CAD build for the part. Positions are in the model's coordinates, mm. Round coordinates to 2 decimals unless told otherwise and drop trailing zeros. Loops run counter-clockwise (first coordinate to the right, second up) from the corner with the lowest first, then second, coordinate; pieces in that order, holes last. Notation, with made-up numbers: (-20, -0.75) -> (5, -0.75) arc R28 cw to (5, 32.25) -> close; hole circle Ø3 at (85.25, 25.25). An arc over 180 degrees is marked (long way). Answer as CSV lines item,"result".
```python
from build123d import *

# Parameters (mm, degrees)
SKETCH1_R           = 12.7
SKETCH1_R_2         = 11.7
EXTRUDE_THIN1_DEPTH = 275.4


with BuildPart() as part:
    # Sketch1 → Extrude-Thin1 (new, symmetric)
    with BuildSketch(Plane(origin=(0, 0, 0), x_dir=(0, 0, -1), z_dir=(1, 0, 0))):
        Circle(SKETCH1_R)
        Circle(SKETCH1_R_2, mode=Mode.SUBTRACT)
    extrude(amount=EXTRUDE_THIN1_DEPTH, both=True)

    # SurfaceCut1
    split(bisect_by=Plane(origin=(131.35, -131.35, 0), x_dir=(-0.7071067811865472, -0.7071067811865478, 0), z_dir=(-0.7071067811865478, 0.7071067811865472, 0)), keep=Keep.TOP)

    # SurfaceCut2
    split(bisect_by=Plane(origin=(-131.35, -131.35, 0), x_dir=(0.7071067811865515, -0.7071067811865436, 0), z_dir=(-0.7071067811865436, -0.7071067811865515, 0)), keep=Keep.BOTTOM)


solid = part.part
```
Q1. Two-plate mould, pull along Y, no slides. Class faces 1 (the cylindrical face through (3.86, -12.4, 2.75)), 2 (the cylindrical face through (-3.84, -11.42, 2.54)), 3 (the flat face through (-262.8, 0.1, -12.2)): pulls with the +Y half, pulls with the -Y half, needs draft (parallel to the pull), parting line crosses it, or undercut.
Results:
face 1,"parting line crosses it"
face 2,"undercut"
face 3,"pulls with the -Y half"
Q2. Slice it at A-A, the plane y = 0. Give the cut face in (x, z).
Results:
outline,"(-262.7, -12.7) -> (262.7, -12.7) -> (262.7, -11.7) -> (-262.7, -11.7) -> close; (-262.7, 11.7) -> (262.7, 11.7) -> (262.7, 12.7) -> (-262.7, 12.7) -> close"
Q3. Slice it at B-B, the plane z = 5.5. Give the cut face in (x, y), and give its area (3 significant figures).
Results:
outline,"(-274.15, 11.45) -> (-273.03, 10.33) -> (273.03, 10.33) -> (274.15, 11.45) -> close; (-252.37, -10.33) -> (-251.25, -11.45) -> (251.25, -11.45) -> (252.37, -10.33) -> close"
area,"1,180 mm2"
Q4. Drop flat-ended pins along their axis: pin 1 Ø5 at (x, y) = (-159.5, -5) entering from +Z; pin 2 Ø10 at (x, z) = (-119, -6) entering from -Y; pin 3 Ø1.5 at (x, z) = (152, -8.5) entering from -Y. Give the stop position or say it passes through.
Results:
pin 1,"z = 12.45"
pin 2,"y = -12.66"
pin 3,"y = -10.06"
Q5. Slice it at C-C, the plane x = 28. Give the cut face in (y, z).
Results:
outline,"circle Ø25.4 at (0, 0); hole circle Ø23.4 at (0, 0)"
Q6. Probe L1, parallel to Z at x = 88, y = 0; L2, parallel to Z at x = 141, y = -1.25. List the from-to ranges inside material, lowest first. Write a range as [from, to].
Results:
L1,"[-12.7, -11.7], [11.7, 12.7]"
L2,"[-12.64, -11.63], [11.63, 12.64]"
